Print and shaded views of the part. All mm, measured from the part's lowest x, y and z. Coordinates: 2 decimals unless noted, no trailing zeros. Write each loop counter-clockwise with the first axis right and the second up, starting at its lowest first coordinate (ties: lowest second). Pieces come first, ordered by that corner, then holes. Notation, with made-up numbers: (45.5, 5) -> (85.5, 5) arc R23 cw to (85.5, 29) -> close; hole circle Ø10 at (11.5, 13). An arc over 180 degrees is marked (long way). Write item = value, one per line.
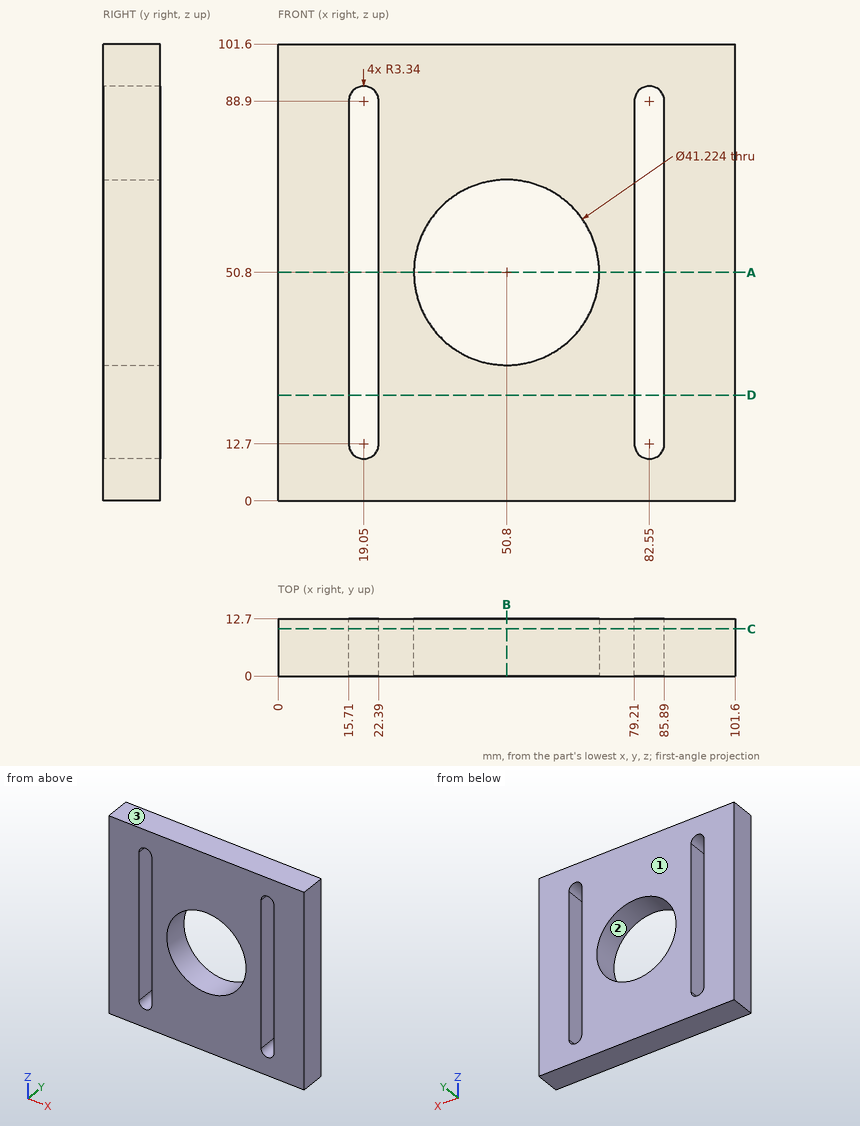
Q1. Probe line 1 (X direction, y = 9.5, z = 88.5); line 2 (Z direction, x = 50.8, y = 9.5); line 3 (X direction, y = 7, z = 49). List the from-to ranges inside material, lowest first. Write a range as from..to.
Model answer:
line_1 = 0..15.71, 22.39..79.21, 85.89..101.6
line_2 = 0..30.19, 71.41..101.6
line_3 = 0..15.71, 22.39..30.27, 71.33..79.21, 85.89..101.6
Q2. Saw through at C-C on y = 10.5. Give the cut face in (x, z).
Model answer:
outline = (0, 0) -> (101.6, 0) -> (101.6, 101.6) -> (0, 101.6) -> close; hole (15.71, 12.7) arc R3.34 ccw to (22.39, 12.7) -> (22.39, 88.9) arc R3.34 ccw to (15.71, 88.9) -> close; hole circle Ø41.22 at (50.8, 50.8); hole (79.21, 12.7) arc R3.34 ccw to (85.89, 12.7) -> (85.89, 88.9) arc R3.34 ccw to (79.21, 88.9) -> close
Q3. Saw through at A-A on z = 50.8. Give the cut face in (x, y).
Model answer:
outline = (0, 0) -> (15.71, 0) -> (15.71, 12.7) -> (0, 12.7) -> close; (22.39, 0) -> (30.19, 0) -> (30.19, 12.7) -> (22.39, 12.7) -> close; (71.41, 0) -> (79.21, 0) -> (79.21, 12.7) -> (71.41, 12.7) -> close; (85.89, 0) -> (101.6, 0) -> (101.6, 12.7) -> (85.89, 12.7) -> close
Q4. Mould opens along Z. For the marked faces 1, 2 and 3 say: released by +Z, released by -Z, zero draft, split by the parting line, or undercut.
Model answer:
face_1 = zero draft
face_2 = undercut
face_3 = released by +Z
Q5. Saw through at D-D on z = 23.5. Give the cut face in (x, y), and give its area (3 significant figures).
Model answer:
outline = (0, 0) -> (15.71, 0) -> (15.71, 12.7) -> (0, 12.7) -> close; (22.39, 0) -> (79.21, 0) -> (79.21, 12.7) -> (22.39, 12.7) -> close; (85.89, 0) -> (101.6, 0) -> (101.6, 12.7) -> (85.89, 12.7) -> close
area = 1,120 mm²
Q6. Saw through at B-B on x = 50.8. Give the cut face in (y, z).
Model answer:
outline = (0, 0) -> (12.7, 0) -> (12.7, 30.19) -> (0, 30.19) -> close; (0, 71.41) -> (12.7, 71.41) -> (12.7, 101.6) -> (0, 101.6) -> close
